The figure shows three views and two pictorial views of one solid part (mm, origin at its lowest corner). Answer the questions. Give positions to 0.01 mm unless a question says otherwise; leave off trailing zeros. Order: outer loops, then holes, each group sorted by start corner. A loop starts at its lowest first (then second) coordinate and runs counter-clockwise, first axis right, second up. Notation, with made-up numbers: (-34, 78.25) - (3, 78.25) arc R23 ccw to (3, 87.25) - close; hole circle Ø7 at (17.25, -12.75). An arc over 180 degrees is marked (long way). Write item = value, one per line.
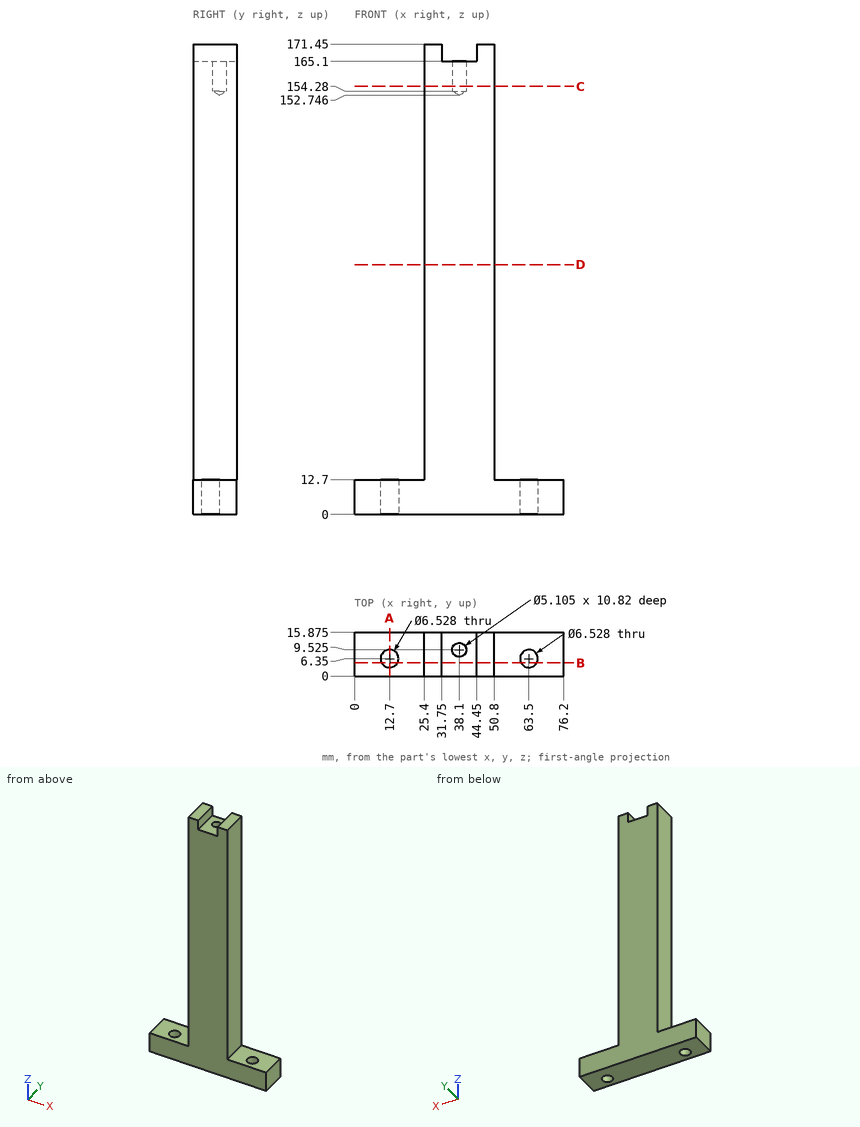
1. Straight lines are drawn through the part: L1, parallel to Z at x = 52, y = 5; L2, parallel to Z at x = 32.5, y = 3; L3, parallel to X at y = 14.75, z = 119. For each, find the intervals that lie inside material, in ascending order. Write a range as [from, to].
Recorded:
L1 = [0, 12.7]
L2 = [0, 165.1]
L3 = [25.4, 50.8]
2. Section C-C (z = 156) is taken. Determine the outline of the cut face in (x, y) (1 decimal), and give its area (3 significant figures).
Recorded:
outline = (25.4, 0) - (50.8, 0) - (50.8, 15.9) - (25.4, 15.9) - close; hole circle Ø5.1 at (38.1, 9.5)
area = 383 mm^2
3. Section D-D (z = 91) is taken. Determine the outline of the cut face in (x, y) (1 decimal).
Recorded:
outline = (25.4, 0) - (50.8, 0) - (50.8, 15.9) - (25.4, 15.9) - close
4. Section B-B (y = 4.75) is taken. Count the separate pieces of the cut face and the enclosed holes in it.
Recorded:
separate_pieces = 3
enclosed_holes = 0
5. Section A-A (x = 12.7) is taken. Determine the outline of the cut face in (y, z) (1 decimal), and give its area (3 significant figures).
Recorded:
outline = (0, 0) - (3.1, 0) - (3.1, 12.7) - (0, 12.7) - close; (9.6, 0) - (15.9, 0) - (15.9, 12.7) - (9.6, 12.7) - close
area = 119 mm^2
6. Flat-ended cylindrical pins translate along their axes: pin 1 (7 mm diameter, centred on y = 8.5, z = 168.5, fed in from -X); pin 2 (3 mm diameter, centred on x = 60.5, y = 2, fed in from +Z); pin 3 (5 mm diameter, centred on y = 9.5, z = 167, fed in from +X). Find the tip coordinate at first contact, or state that the pin passes through.
Recorded:
pin_1 = 25.4
pin_2 = 12.7
pin_3 = 50.8
